Autodesk Inventor part; units mm, degrees
ref_plane "YZ Plane" through (0, 0, 0) normal (1, 0, 0) x (0, 1, 0)
ref_plane "XZ Plane" through (0, 0, 0) normal (0, 1, 0) x (-1, 0, 0)
ref_plane "XY Plane" through (0, 0, 0) normal (0, 0, 1) x (1, 0, 0)
sketch "Sketch1" plane through (0, 0, 0) normal (0, 1, 0) x (-1, 0, 0)
  line L0 (50, -50) -> (-50, -50)
  line L1 (-50, -50) -> (-50, 50)
  line L2 (-50, 50) -> (50, 50)
  line L3 (50, 50) -> (50, -50)
  point P0 (0, 0)
  point P1 (0, 0)
  dimension "d0" = 100
  dimension "d1" = 100
  dimension "d2" = 50
extrude "Extrusion1" add sketch "Sketch1" along normal blind 95
sketch "Sketch2" plane through (0, 95, 0) normal (0, 1, 0) x (1, 0, 0)
  line L0 (-45, 45) -> (45, 45)
  line L1 (45, 45) -> (45, -45)
  line L2 (45, -45) -> (-45, -45)
  line L3 (-45, -45) -> (-45, 45)
  line L4 (50, -50) -> (50, 50)
  line L5 (-50, 50) -> (-50, -50)
  line L6 (-50, -50) -> (50, -50)
  line L7 (-50, 50) -> (50, 50)
  point P0 (0, 0)
  dimension "d5" = 5
  dimension "d6" = 5
  dimension "d7" = 5
  dimension "d8" = 5
extrude "Extrusion2" cut sketch "Sketch2" against normal blind 85 contours L0 L1 L2 L3
sketch "Sketch3" plane through (0, 95, 0) normal (0, 1, 0) x (1, 0, 0)
  line L0 (50, -50) -> (50, 50)
  circle A0 centre (47.5, 47.5) radius 1
  line L1 (-50, 50) -> (50, 50)
  line L2 (-50, -50) -> (50, -50)
  circle A1 centre (47.5, -47.5) radius 1
  line L3 (-50, 50) -> (-50, -50)
  circle A2 centre (-47.5, -47.5) radius 1
  circle A3 centre (-47.5, 47.5) radius 1
  point P0 (0, 0)
  point P1 (47.5, -47.5)
  dimension "d12" = 2.5
  dimension "d13" = 2.5
  dimension "d14" = 2.5
  dimension "d15" = 2.5
  dimension "d16" = 2
  dimension "d17" = 2.5
  dimension "d18" = 2.5
  dimension "d19" = 2.5
  dimension "d20" = 2.5
hole "Hole2" at (47.5, 95, -47.5) at (47.5, 95, 47.5) at (-47.5, 95, 47.5) at (-47.5, 95, -47.5) direction (0, -1, 0) diameter 2 depth 8
sketch "Sketch9" plane through (-45, 95, 45) normal (1, 0, 0) x (0, 0, -1)
  circle A0 centre (45, -45) radius 10.5
  point P0 (45, -95)
  dimension "d66" = 21
extrude "Extrusion4" cut sketch "Sketch9" against normal blind 3
sketch "Sketch10" plane through (0, 10, 0) normal (0, 1, 0) x (1, 0, 0)
  circle A0 centre (0, 0) radius 10.5
  dimension "d69" = 21
extrude "Extrusion5" cut sketch "Sketch10" against normal blind 3
sketch "Sketch11" plane through (45, 95, 45) normal (0, 0, -1) x (-1, 0, 0)
  circle A0 centre (45, -45) radius 10.5
  line L0 (0, 0) -> (0, -85)
  line L1 (0, 0) -> (90, 0)
  point P0 (45, -95)
  dimension "d72" = 45
  dimension "d73" = 45
  dimension "d74" = 21
extrude "Extrusion6" cut sketch "Sketch11" against normal blind 3
sketch "Sketch13" plane through (0, 50, 48) normal (0, 0, -1) x (-1, 0, 0)
  circle A0 centre (0, 0) radius 1.75
  point P0 (0, -50)
  dimension "d77" = 3.5
properties part number "cubesat"
Geometry check sheet. Reference: the model listing, model coordinates, mm. A direction names the side the tool comes from. Give positions to 0.01 mm unless a question says otherwise; leave off trailing zeros. Order: outer loops, then holes, each group sorted by start corner. A loop starts at its lowest first (then second) coordinate and runs counter-clockwise, first axis right, second up. Notation, with made-up numbers: (65, 19) -> (79, 19) arc R18 ccw to (79, 23) -> close; hole circle Ø8 at (6.5, 37). An arc over 180 degrees is marked (long way). Write each question's results on one line, items separated by ' | '. Start each with the question number.
(1) Sectioned sample at C-C (x = 0). Enter the section's corners in (y, z).
(2) Mould release check, pull along Y, two halves, no side actions. Record for faces 1 (the face through (-4.845, 40.685, 46.479)), 2 (the face through (-46.479, 40.685, -4.845)), 3 (the face through (50, 47, -1)), 4 (the face through (-1, 10, -11)): pulls with the +Y half, pulls with the -Y half, needs draft (parallel to the pull), parting line crosses it, or undercut.
(3) Sectioned sample at A-A (y = 50). Enter the section's corners in (x, z).
(4) Sectioned sample at D-D (y = 31). Enter the section's corners in (x, z).
(5) Sectioned sample at B-B (z = 35). Enter the section's corners in (x, y), plus the area to 3 significant figures.
(6) Gauge pin test, flat ends, axial feed: P1, Ø1.2, axis at x = 47.5, z = 47.5, coming from the +Y side; P2, Ø3, axis at x = 13.5, z = 19, coming from the +Y side; P3, Ø1, axis at x = -48, z = 48, coming from the +Y side. Record the tip position at first contact, or that the pin passes through.
(7) Scan lines: line 1 (X direction, y = 90.5, z = 47.5); line 2 (X direction, y = 21.5, z = 23). Record each from-to range of solid material in increasing order.
(8) Access from +Z, -Z, +X, -X, +Y, -Y to the whole of each face (thin tool, end or side, straight path). Record for faces 5 (the face through (-45, 63, 1)), 6 (the face through (-1, 47, -50)), 7 (the face through (-48, 50, 0)).
Answer below:
1) outline: (0, -50) -> (95, -50) -> (95, -45) -> (10, -45) -> (10, -10.5) -> (7, -10.5) -> (7, 10.5) -> (10, 10.5) -> (10, 45) -> (39.5, 45) -> (39.5, 48) -> (60.5, 48) -> (60.5, 45) -> (95, 45) -> (95, 50) -> (0, 50) -> close
2) face 1: undercut | face 2: undercut | face 3: needs draft | face 4: pulls with the +Y half
3) outline: (-50, -50) -> (50, -50) -> (50, 50) -> (-50, 50) -> close; hole (-48, -10.5) -> (-45, -10.5) -> (-45, -45) -> (45, -45) -> (45, 45) -> (10.5, 45) -> (10.5, 48) -> (-10.5, 48) -> (-10.5, 45) -> (-45, 45) -> (-45, 10.5) -> (-48, 10.5) -> close
4) outline: (-50, -50) -> (50, -50) -> (50, 50) -> (-50, 50) -> close; hole (-45, -45) -> (45, -45) -> (45, 45) -> (-45, 45) -> close
5) outline: (-50, 0) -> (50, 0) -> (50, 95) -> (45, 95) -> (45, 10) -> (-45, 10) -> (-45, 95) -> (-50, 95) -> close | area: 1,850 mm2
6) P1: y = 87 | P2: y = 10 | P3: y = 95
7) line 1: -50 to -48.5, -46.5 to 46.5, 48.5 to 50 | line 2: -50 to -45, 45 to 50
8) face 5: +Y | face 6: -Z, +X, -X, +Y, -Y | face 7: none
